CAD build for the part. Positions are in the model's coordinates, mm. A direction names the side the tool comes from. Give positions to 0.01 mm unless a question says otherwise; leave off trailing zeros. Loops run counter-clockwise (first coordinate to the right, second up) from the corner with the lowest first, then second, coordinate; pieces in that order, holes last. Notation, with made-up numbers: M 35,65 L 59,65 A12 ccw 59,88 Z; hole C -17,-9 d9. An arc over 180 degrees is marked long. One line per question, with ' | ' between items.
```python
from build123d import *

# Parameters (mm, degrees)
PAD_DEPTH       = 6
SKETCH002_R     = 4.5
SKETCH002_R_2   = 1.3
POCKET001_DEPTH = 20
SKETCH005_R     = 1.8
POCKET_DEPTH    = 5
SKETCH006_R     = 1.8
POCKET002_DEPTH = 6
CHAMFER_SIZE    = 1


with BuildPart() as part:
    # Sketch → Pad (new body)
    with BuildSketch(Plane.XY):
        Polygon((0, 20), (0, -20), (0, -28), (4, -28), (4, -20), (32, -20), (32, 20), (4, 20), (4, 28), (0, 28), align=None)
    extrude(amount=PAD_DEPTH)

    # Sketch002 → Pocket001 (cut)
    with BuildSketch(Plane.XY.offset(6)):
        with Locations((16, 0)):
            Circle(SKETCH002_R)
        with Locations((16, 8)):
            Circle(SKETCH002_R_2)
        with Locations((21.656854, 5.656854)):
            Circle(SKETCH002_R_2)
        with Locations((24, 0)):
            Circle(SKETCH002_R_2)
        with Locations((21.656854, -5.656854)):
            Circle(SKETCH002_R_2)
        with Locations((16, -8)):
            Circle(SKETCH002_R_2)
        with Locations((10.343146, -5.656854)):
            Circle(SKETCH002_R_2)
        with Locations((8, 0)):
            Circle(SKETCH002_R_2)
        with Locations((10.343146, 5.656854)):
            Circle(SKETCH002_R_2)
    extrude(amount=-POCKET001_DEPTH, mode=Mode.SUBTRACT)

    # Sketch005 → Pocket (cut)
    with BuildSketch(Plane(origin=(0, 0, 0), x_dir=(0, -1, 0), z_dir=(-1, 0, 0))):
        with Locations((23, 3)):
            Circle(SKETCH005_R)
        with Locations((-23, 3)):
            Circle(SKETCH005_R)
    extrude(amount=-POCKET_DEPTH, mode=Mode.SUBTRACT)

    # Sketch006 (on Face4 of Pocket) → Pocket002 (cut)
    with BuildSketch(Plane(origin=(0, 0, 0), x_dir=(1, 0, 0), z_dir=(0, 0, -1))):
        with Locations((25, 16)):
            Circle(SKETCH006_R)
        with Locations((25, -16)):
            Circle(SKETCH006_R)
    extrude(amount=-POCKET002_DEPTH, mode=Mode.SUBTRACT)

    # Chamfer
    chamfer_edges = [part.edges().sort_by_distance(p)[0] for p in [
        (20.356854, -5.656854, 6),
        (22.7, 0, 6),
        (20.356854, 5.656854, 6),
        (14.7, 8, 6),
        (9.043146, 5.656854, 6),
        (6.7, 0, 6),
        (9.043146, -5.656854, 6),
        (14.7, -8, 6),
    ]]
    chamfer(chamfer_edges, length=CHAMFER_SIZE)


solid = part.part
```
Item 1: Saw through at A-A on y = 16. Give the cut face in (x, z), and give its area (3 significant figures).
Conclusion:
outline: M 0,0 L 23.2,0 L 23.2,6 L 0,6 Z; M 26.8,0 L 32,0 L 32,6 L 26.8,6 Z | area: 170 mm²
Item 2: Saw through at B-B on z = 3. State how many separate pieces and enclosed holes the cut face has, and give its area (3 significant figures).
Conclusion:
separate pieces: 3 | enclosed holes: 11 | area: 1,190 mm²
Item 3: Mould opens along Y. For faces 4 (the cylindrical face through (11.544, 5.159, 2.535)), 5 (the flat face through (2, -28, 3)), 6 (the cylindrical face through (22.7, 0.06, 2.54)), 7 (the flat face through (32, 0, 3)) say: pulls with the +Y half, pulls with the -Y half, needs draft (parallel to the pull), parting line crosses it, or undercut.
Conclusion:
face 4: undercut | face 5: pulls with the -Y half | face 6: undercut | face 7: needs draft
Item 4: Drop flat-ended pins along their axis: P1, Ø2.5, axis at x = 21.66, y = 5.66, coming from the -Z side; P2, Ø3.5, axis at x = 24, y = 0, coming from the +Z side; P3, Ø4, axis at x = 16, y = 8, coming from the +Z side; P4, Ø2, axis at x = 8, z = 2.5, coming from the +Y side. Give the stop position or say it passes through.
Conclusion:
P1: through | P2: z = 5.45 | P3: z = 5.7 | P4: y = 20
Item 5: Saw through at D-D on y = 23. Give the cut face in (x, z).
Conclusion:
outline: M 0,0 L 4,0 L 4,1.2 L 0,1.2 Z; M 0,4.8 L 4,4.8 L 4,6 L 0,6 Z
Item 6: Saw through at C-C on x = 16. Give the cut face in (y, z).
Conclusion:
outline: M -20,0 L -9.3,0 L -9.3,5 L -10.3,6 L -20,6 Z; M -6.7,0 L -4.5,0 L -4.5,6 L -5.7,6 L -6.7,5 Z; M 4.5,0 L 6.7,0 L 6.7,5 L 5.7,6 L 4.5,6 Z; M 9.3,0 L 20,0 L 20,6 L 10.3,6 L 9.3,5 Z
Item 7: Drill centre lines: line 1 along Y through (x, z) = (16, 2.85); line 2 along X through (y, z) = (0.5, 0.5); line 3 along X through (y, z) = (1, 2.3). Where is each one in solid material? Low to high. Write a range as [from, to].
Conclusion:
line 1: [-20, -9.3], [-6.7, -4.5], [4.5, 6.7], [9.3, 20] | line 2: [0, 6.8], [9.2, 11.53], [20.47, 22.8], [25.2, 32] | line 3: [0, 7.17], [8.83, 11.61], [20.39, 23.17], [24.83, 32]
Item 8: 3-axis set-ups, long thin cutter, end or side, ignore diameter. For faces 1 (the cylindrical face through (22.86, -6.15, 2.54)), 2 (the flat face through (4, 25, 3)), 3 (the flat face through (4, -25, 3)): which of +Z, -Z, +X, -X, +Y, -Y reach the whole face in a straight line?
Conclusion:
face 1: +Z, -Z | face 2: +Z, -Z, +X, +Y | face 3: +Z, -Z, +X, -Y
